Verification items for this drawing (mm, ordinates from the low corner). A direction names the side the tool comes from. Give positions to 0.01 mm unless a question says otherwise; leave off trailing zeros. Loops run counter-clockwise (first coordinate to the right, second up) from the corner with the lowest first, then second, coordinate; pieces in that order, holes last. Notation, with made-up numbers: (48.5, -24) -> (85.5, -24) arc R8 cw to (85.5, -13) -> close; hole circle Ø1 at (33.25, -30.75). An arc over 180 degrees is marked (long way). Write item = value, one per line.
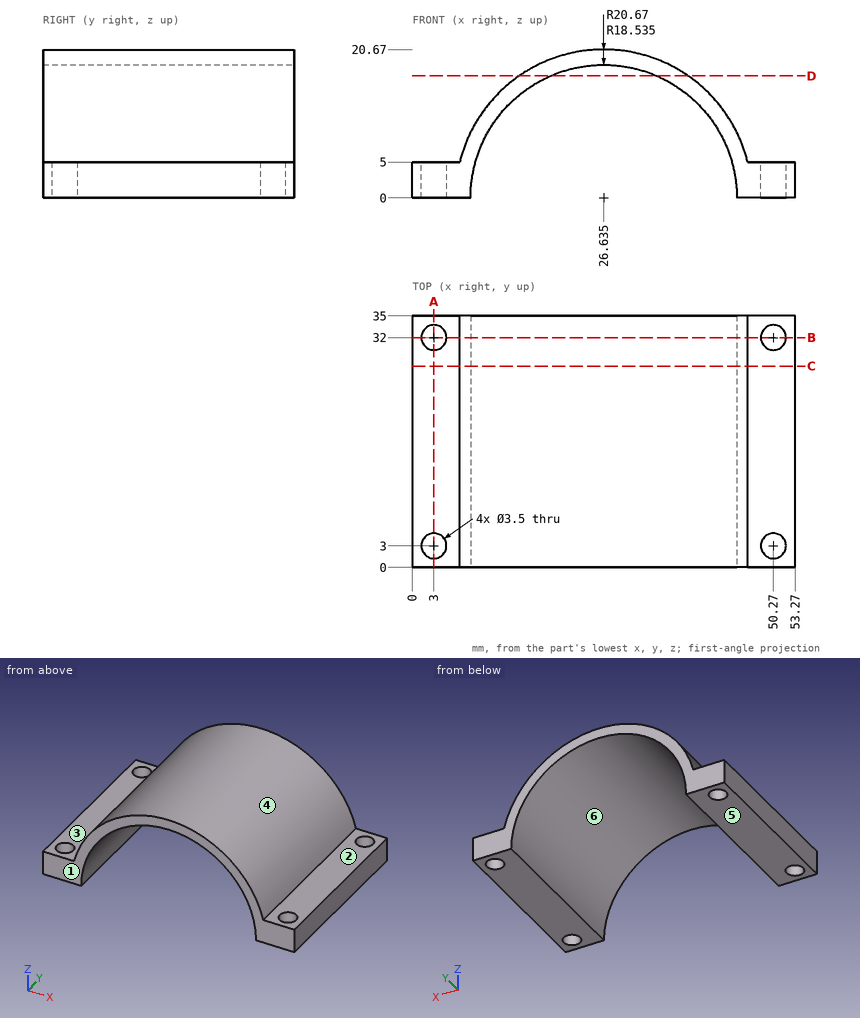
Item 1: Section check A-A, the plane x = 3. Record the cut outline in (y, z), plus the area to 3 significant figures.
Answer:
outline = (0, 0) -> (1.25, 0) -> (1.25, 5) -> (0, 5) -> close; (4.75, 0) -> (30.25, 0) -> (30.25, 5) -> (4.75, 5) -> close; (33.75, 0) -> (35, 0) -> (35, 5) -> (33.75, 5) -> close
area = 140 mm^2
Item 2: Section check C-C, the plane y = 28. Record the cut outline in (x, z) (3 decimals), plus the area to 3 significant figures.
Answer:
outline = (0, 0) -> (8.1, 0) arc R18.535 cw to (45.17, 0) -> (53.27, 0) -> (53.27, 5) -> (46.691, 5) arc R20.67 ccw to (6.579, 5) -> (0, 5) -> close
area = 193 mm^2
Item 3: Draft check along X on the marked faces 4, 5 and 6. Enter one of: +X half, -X half, draft (parallel to the pull), parting line (faces both ways), or undercut.
Answer:
face_4 = parting line
face_5 = draft
face_6 = undercut
Item 4: Tool access check on the marked faces 1, 2 and 3. Record the directions out of +Z, -Z, +X, -X, +Y, -Y that give a thin tool (end or side, any length) a straight path to the whole face; none if there is none.
Answer:
face_1 = +Z, -Z, +X, -X, -Y
face_2 = +Z, +X, +Y, -Y
face_3 = +Z, -X, +Y, -Y
Item 5: Thickness scan on L1, parallel to Y at x = 50.27, z = 1.95; L2, parallel to X at y = 3, z = 2.65; L3, parallel to Z at x = 3.5, y = 25.5. Record the ranges inside material, lowest first. Write a range as [from, to].
Answer:
L1 = [0, 1.25], [4.75, 30.25], [33.75, 35]
L2 = [0, 1.25], [4.75, 8.29], [44.98, 48.52], [52.02, 53.27]
L3 = [0, 5]
Item 6: Gauge pin test, flat ends, axial feed: pin 1 (2 mm diameter, centred on x = 2, y = 22.5, fed in from +Z); pin 2 (2 mm diameter, centred on x = 3, y = 3, fed in from +Z); pin 3 (6 mm diameter, centred on y = 16, z = 18.5, fed in from -X); pin 4 (6 mm diameter, centred on y = 21.5, z = 17.5, fed in from -X). Record the tip position at first contact, or that the pin passes through.
Answer:
pin_1 = 5
pin_2 = through
pin_3 = 12.96
pin_4 = 11.9
Item 7: Section check B-B, the plane y = 32. Record the cut outline in (x, z) (3 decimals), plus the area to 3 significant figures.
Answer:
outline = (0, 0) -> (1.25, 0) -> (1.25, 5) -> (0, 5) -> close; (4.75, 0) -> (8.1, 0) arc R18.535 cw to (45.17, 0) -> (48.52, 0) -> (48.52, 5) -> (46.691, 5) arc R20.67 ccw to (6.579, 5) -> (4.75, 5) -> close; (52.02, 0) -> (53.27, 0) -> (53.27, 5) -> (52.02, 5) -> close
area = 158 mm^2
Item 8: Section check D-D, the plane z = 17. Record the cut outline in (x, y), plus the area to 3 significant figures.
Answer:
outline = (14.88, 0) -> (19.25, 0) -> (19.25, 35) -> (14.88, 35) -> close; (34.02, 0) -> (38.39, 0) -> (38.39, 35) -> (34.02, 35) -> close
area = 306 mm^2
